from build123d import *

# Parameters (mm, degrees)
SKETCH1_R                = 10.85
BOSS_EXTRUDE1_DEPTH      = 1
SKETCH2_R                = 4.9
BOSS_EXTRUDE2_DEPTH      = 5
SKETCH3_R                = 3.9
BOSS_EXTRUDE3_DEPTH      = 4.5
SKETCH4_R                = 1.5
BOSS_EXTRUDE4_DEPTH      = 4.5
CHAMFER1_SIZE            = 1
SKETCH5_R                = 3.1
CUT_EXTRUDE1_DEPTH       = 7.5
CUT_EXTRUDE_THIN2_START  = -0.4
SKETCH6_W                = 2
SKETCH6_H                = 21.149646587
CUT_EXTRUDE_THIN2_DEPTH  = 22.857982198
CIRPATTERN1_COUNT        = 4
SKETCH8_R                = 5.669003214
SKETCH8_R_2              = 4.883775851
BOSS_EXTRUDE5_DEPTH      = 1
SKETCH10_R               = 6.62346743
SKETCH10_R_2             = 4.788629078
BOSS_EXTRUDE6_DEPTH      = 0.1
SWEEP1_START             = -2.295822316
SWEEP1_DEPTH             = 4.591644632
EXTRUDE_THIN1_DEPTH      = 8
EXTRUDE_THIN1_DEPTH_BACK = 4
SKETCH13_R               = 2.5
SKETCH13_R_2             = 1.5


# Read off the part's stored shape, not the designer's step: Sweep1
with BuildPart() as part:
    # Sketch1 → Boss-Extrude1 (new body)
    with BuildSketch(Plane(origin=(0, 0, 0), x_dir=(1, 0, 0), z_dir=(0, 1, 0))):
        with Locations(Location((0, 0, 0), (0, 0, 270))):
            Circle(SKETCH1_R)
    extrude(amount=BOSS_EXTRUDE1_DEPTH)

    # Sketch2 → Boss-Extrude2 (add)
    with BuildSketch(Plane.XZ):
        with Locations(Location((0, 0, 0), (0, 0, 270))):
            Circle(SKETCH2_R)
    extrude(amount=BOSS_EXTRUDE2_DEPTH)

    # Sketch3 → Boss-Extrude3 (add)
    with BuildSketch(Plane.XZ.offset(5)):
        with Locations(Location((0, 0, 0), (0, 0, 270))):
            Circle(SKETCH3_R)
    extrude(amount=BOSS_EXTRUDE3_DEPTH)

    # Sketch4 → Boss-Extrude4 (add)
    with BuildSketch(Plane.XZ.offset(9.5)):
        with Locations(Location((0, 0, 0), (0, 0, 270))):
            Circle(SKETCH4_R)
    extrude(amount=BOSS_EXTRUDE4_DEPTH)

    # Chamfer1
    chamfer1_edges = [part.edges().sort_by_distance(p)[0] for p in [
        (0, 0, 4.9),
    ]]
    chamfer(chamfer1_edges, length=CHAMFER1_SIZE)

    # Sketch5 → Cut-Extrude1 (cut)
    with BuildSketch(Plane(origin=(0, 1, 0), x_dir=(1, 0, 0), z_dir=(0, 1, 0))):
        with Locations(Location((0, 0, 0), (0, 0, 270))):
            Circle(SKETCH5_R)
    extrude(amount=-CUT_EXTRUDE1_DEPTH, mode=Mode.SUBTRACT)

    # Sketch6 → Cut-Extrude-Thin2 (cut)
    with BuildSketch(Plane(origin=(0, 1, 0), x_dir=(1, 0, 0), z_dir=(0, 1, 0)).offset(CUT_EXTRUDE_THIN2_START)):
        with Locations((0, 10.574823294)):
            Rectangle(SKETCH6_W, SKETCH6_H)
    cut_extrude_thin2 = extrude(amount=CUT_EXTRUDE_THIN2_DEPTH, mode=Mode.SUBTRACT)

    # CirPattern1: Cut-Extrude-Thin2 ×4 about axis
    cirpattern1_axis = Axis((0, 0, 0), (0, 1, 0))
    for i in range(1, CIRPATTERN1_COUNT):
        add(cut_extrude_thin2.rotate(cirpattern1_axis, i * 360 / CIRPATTERN1_COUNT), mode=Mode.SUBTRACT)

    # Sketch8 → Boss-Extrude5 (add)
    with BuildSketch(Plane(origin=(0, -1, 0), x_dir=(-1, 0, 0), z_dir=(0, -1, 0))):
        with Locations(Location((0, 0, 0), (0, 0, 90))):
            Circle(SKETCH8_R)
        Circle(SKETCH8_R_2, mode=Mode.SUBTRACT)
    extrude(amount=BOSS_EXTRUDE5_DEPTH)



with BuildPart() as body_2:
    # Sketch10 → Boss-Extrude6 (new body)
    with BuildSketch(Plane(origin=(0, -1, 0), x_dir=(1, 0, 0), z_dir=(0, 1, 0))):
        with Locations(Location((0, 0, 0), (0, 0, 270))):
            Circle(SKETCH10_R)
        with Locations(Location((0, 0, 0), (0, 0, 270))):
            Circle(SKETCH10_R_2, mode=Mode.SUBTRACT)
    extrude(amount=BOSS_EXTRUDE6_DEPTH)

    # Sweep1 outline → Sweep1 (add)
    with BuildSketch(Plane.XY.offset(SWEEP1_START)):
        with BuildLine():
            Line((6.894755274, -1), (6.352179586, -1))
            add(Edge.make_bspline(
                [(6.352179586, -1), (8.215144945, -3.590953031), (9.19411107, -6.50188171), (9.289077959, -9.732786039)],
                knots=[0, 0, 0, 0, 1, 1, 1, 1], degree=3))
            Line((9.289077959, -9.732786039), (9.831653647, -9.732786039))
            add(Edge.make_bspline(
                [(6.894755274, -1), (8.757720633, -3.590953031), (9.736686757, -6.50188171), (9.831653647, -9.732786039)],
                knots=[0, 0, 0, 0, 1, 1, 1, 1], degree=3))
        make_face()
    extrude(amount=SWEEP1_DEPTH)


with BuildPart() as part_1:
    add(part.part)

    add(body_2.part)  # Extrude-Thin1 merges body 2
    # Sketch13 → Extrude-Thin1 (add, two sides: drawn at the far end of the back side and taken through both)
    with BuildSketch(Plane.XZ.offset(9.732786039).offset(-EXTRUDE_THIN1_DEPTH_BACK)):
        with Locations((6.789077959, 0)):
            Circle(SKETCH13_R)
        with Locations((6.789077959, 0)):
            Circle(SKETCH13_R_2, mode=Mode.SUBTRACT)
    extrude(amount=EXTRUDE_THIN1_DEPTH + EXTRUDE_THIN1_DEPTH_BACK)


solid = part_1.part
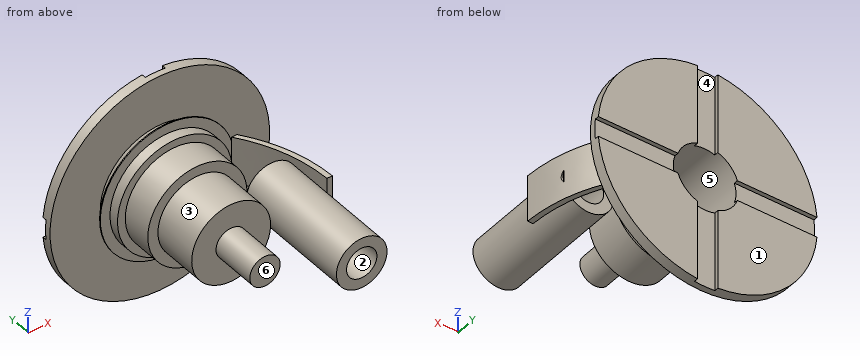
Read the model definition and answer for the solid it produces. Units are mm, in the model's axes. Face numbers are marked on the shaded views. A direction names the side the tool comes from. Round coordinates to 2 decimals unless told otherwise and drop trailing zeros. Loops run counter-clockwise (first coordinate to the right, second up) from the corner with the lowest first, then second, coordinate; pieces in that order, holes last.
Q1. Section C-C on z = 7.25 is taken. Write down the section's boundary in (x, y), and give its area (3 significant figures).
Q2. Determine the mould class of the marked faces 1, 2 and 3 for opening direction Z: released by +Z, released by -Z, zero draft, split by the parting line, or undercut.
Q3. Each of these flat-tipped pins is pushed along its axis until it touches: pin 1 (2 mm diameter, centred on x = 6.5, y = -3, fed in from +Z); pin 2 (6 mm diameter, centred on x = -3, z = -6.5, fed in from -Y); pin 3 (10 mm diameter, centred on x = -5.5, z = -2, fed in from -Y). Where does it stop, or does it pass through?
Q4. Which of the six approach directions +Z, -Z, +X, -X, +Y, -Y give full straight-line access (tool end or side, diameter ignored) to the marked faces 4, 5 and 6?
Q5. Consider probe 1 along X at (y, z) = (-2.25, 0); probe 2 along Y at (x, z) = (-0.75, 0.5); probe 3 along X at (y, z) = (-7, 2). Determine where each line is inside the solid, lowest interval first.
Q6. Section D-D on z = 9.5 is taken. Write down the section's boundary in (x, y), and give its area (3 significant figures).
Q7. Section B-B on y = -7 is taken. Give the number of separate pieces and of enclosed holes in the cut face, and give its area (3 significant figures).
Output:
1. outline: (-8.07, 0) - (8.07, 0) - (8.07, 1) - (1, 1) - (1, 0.6) - (-1, 0.6) - (-1, 1) - (-8.07, 1) - close
1. area: 15.3 mm2
2. face 1: zero draft
2. face 2: undercut
2. face 3: split by the parting line
3. pin 1: stops at z = 2.3
3. pin 2: stops at y = -5
3. pin 3: stops at y = -14
4. face 4: +Z, -Z, +Y
4. face 5: +Y
4. face 6: +Z, -Z, -X, -Y
5. probe 1: x = -4.9 to -3.1, 3.1 to 4.9, 7.17 to 7.71
5. probe 2: y = -14 to -6.5
5. probe 3: x = -3.35 to 3.35, 5.29 to 8.29, 8.98 to 9.53
6. outline: (-5.24, 0) - (5.24, 0) - (5.24, 1) - (1, 1) - (1, 0.6) - (-1, 0.6) - (-1, 1) - (-5.24, 1) - close
6. area: 9.68 mm2
7. separate pieces: 2
7. enclosed holes: 1
7. area: 62.3 mm2
